Autodesk Inventor part; units mm, degrees
ref_plane "YZ Plane" through (0, 0, 0) normal (1, 0, 0) x (0, 1, 0)
ref_plane "XZ Plane" through (0, 0, 0) normal (0, 1, 0) x (-1, 0, 0)
ref_plane "XY Plane" through (0, 0, 0) normal (0, 0, 1) x (1, 0, 0)
sketch "Sketch1" plane through (0, 0, 0) normal (0, 1, 0) x (-1, 0, 0)
  line L0 (0, 0) -> (33, 0)
  line L1 (71, 0) -> (71, -33)
  line L2 (71, -33) -> (38, -33)
  line L3 (0, -33) -> (0, 0)
  line L4 (0, -33) -> (0, 0)
  line L5 (75, -37) -> (75, 4)
  line L6 (75, 4) -> (-4, 4)
  line L7 (-4, 4) -> (-4, -37)
  line L8 (-4, -37) -> (75, -37)
  line L9 (-10, 10) -> (81, 10)
  line L10 (81, 10) -> (81, -43)
  line L11 (81, -43) -> (-10, -43)
  line L12 (-10, -43) -> (-10, 10)
  line L13 (38, -33) -> (38, 0)
  line L14 (33, -33) -> (33, 0)
  line L15 (38, -33) -> (33, -33)
  line L16 (33, -33) -> (0, -33)
  line L17 (38, 0) -> (71, 0)
  line L18 (33, 0) -> (38, 0)
  point P0 (0, -33)
  point P1 (0, -37)
  point P2 (0, 4)
  dimension "d0" = 33
  dimension "d1" = 71
  dimension "d5" = 4
  dimension "d10" = 6
  dimension "d19" = 33
  dimension "d20" = 33
extrude "Extrusion1" add sketch "Sketch1" along normal blind 6 contours L0 L14 L16 L3 | L18 L13 L15 L14 | L17 L1 L2 L13 | L8 L7 L6 L5 | L9 L10 L11 L12
extrude "Extrusion4" add sketch "Sketch1" along normal blind 66 contours L18 L13 L15 L14 | L8 L7 L6 L5
chamfer "Chamfer3" distance 6 angle 45 4 edges at (-75, 6, -16.5) (-35.5, 6, 4) (4, 6, -16.5) (-35.5, 6, -37)
equation "\"d19\" = d0"
equation "\"d20\" = d19"
properties part number "double"
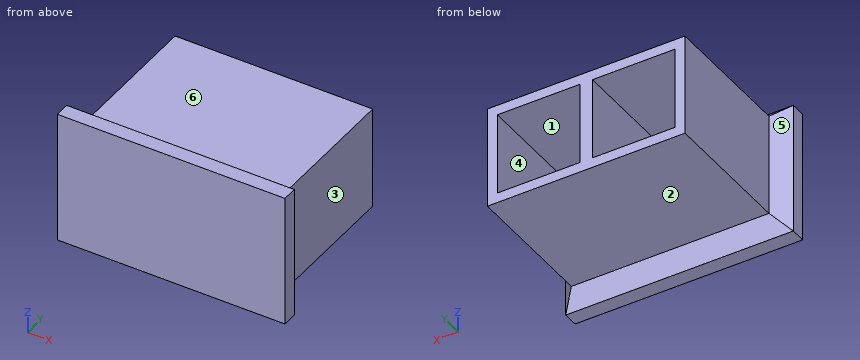
Source: CAD feature listing. Evaluate the final solid. Frame: model axes, mm. Face numbers are marked on the shaded views. A direction names the side the tool comes from. Round coordinates to 2 decimals unless told otherwise and drop trailing zeros. Loops run counter-clockwise (first coordinate to the right, second up) from the corner with the lowest first, then second, coordinate; pieces in that order, holes last. Notation, with made-up numbers: M 17.25,-24.75 L 48.25,-24.75 A6 cw 48.25,-18.75 Z; hole C 71.5,-16 d4. An arc over 180 degrees is marked long. Answer as CSV lines item,"result".
Q1. Pull-direction query (Z, two-part tool) for the marked faces 4, 5 and 6; classes: +Z half, -Z half, draft (parallel to the pull), parting line (faces both ways), or undercut.
Verdict:
face 4,"undercut"
face 5,"draft"
face 6,"+Z half"
Q2. Contact query for flat-ended pins moving along their axis: pin 1 (10 mm diameter, centred on y = 49.5, z = -24, fed in from +X); pin 2 (6 mm diameter, centred on x = -46, y = 45, fed in from -Z); pin 3 (3 mm diameter, centred on x = -46, z = -8.5, fed in from +Y). Output: stop coordinate, or through.
Verdict:
pin 1,"stops at x = 4"
pin 2,"stops at z = -37"
pin 3,"stops at y = 6"
Q3. Reachability of the marked faces 1, 2 and 3 from +Z, -Z, +X, -X, +Y, -Y: full face, straight path, thin tool, end or side. Return the list, or none.
Verdict:
face 1,"+Y"
face 2,"-Z, +X, -X, +Y"
face 3,"+Z, -Z, +X, +Y"
Q4. Line query: line 1 along X through (y, z) = (50, -11.5); line 2 along Z through (x, y) = (-22.5, 26.5); line 3 along X through (y, z) = (10, -7). Output: solid intervals per line, ascending.
Verdict:
line 1,"x = -75 to -71, -38 to -33, 0 to 4"
line 2,"z = -37 to -33, 0 to 4"
line 3,"x = -77 to -71, -38 to -33, 0 to 6"
Q5. Cut plane A-A (y = 51). Return the cut outline in (x, z), plus the area to 3 significant figures.
Verdict:
outline,"M -75,-37 L 4,-37 L 4,4 L -75,4 Z; hole M -71,-33 L -38,-33 L -38,0 L -71,0 Z; hole M -33,-33 L 0,-33 L 0,0 L -33,0 Z"
area,"1,060 mm^2"
